Part model, mm, in its own coordinate system. A direction names the side the tool comes from. Coordinates: 2 decimals unless noted, no trailing zeros. Order: outer loops, then holes, each group sorted by start corner. A loop starts at its lowest first (then second) coordinate and runs counter-clockwise, first axis right, second up.
from build123d import *

# Parameters (mm, degrees)
PAD_DEPTH          = 4
SKETCH001_R        = 22.5
PAD001_DEPTH       = 2
SKETCH002_W        = 1.5
SKETCH002_H        = 5
POCKET_DEPTH       = 129.531389
POLARPATTERN_COUNT = 20


with BuildPart() as part:
    # Sketch → Pad (new body)
    with BuildSketch(Plane.XY):
        Polygon((-6.119913, 10.6), (-12.239826, 0), (-6.119913, -10.6), (6.119913, -10.6), (12.239826, 0), (6.119913, 10.6), align=None)
        Polygon((-4.965212, 8.6), (-9.930425, 0), (-4.965212, -8.6), (4.965212, -8.6), (9.930425, 0), (4.965212, 8.6), align=None, mode=Mode.SUBTRACT)
    extrude(amount=PAD_DEPTH)

    # Sketch001 (on Face13 of Pad) → Pad001 (join)
    with BuildSketch(Plane(origin=(0, 0, 0), x_dir=(1, 0, 0), z_dir=(0, 0, -1))):
        Circle(SKETCH001_R)
        Polygon((-6.119913, 10.6), (-12.239826, 0), (-6.119913, -10.6), (6.119913, -10.6), (12.239826, 0), (6.119913, 10.6), align=None, mode=Mode.SUBTRACT)
    extrude(amount=-PAD001_DEPTH)

    # Sketch002 (on Face2 of Pad001) → Pocket (cut, through all)
    with BuildSketch(Plane.XY.offset(2)):
        with Locations((0, 20)):
            Rectangle(SKETCH002_W, SKETCH002_H)
    pocket = extrude(amount=-POCKET_DEPTH, mode=Mode.SUBTRACT)

    # PolarPattern: Pocket ×20 about axis
    polarpattern_axis = Axis((0, 0, 0), (0, 0, 1))
    for i in range(1, POLARPATTERN_COUNT):
        add(pocket.rotate(polarpattern_axis, i * 360 / POLARPATTERN_COUNT), mode=Mode.SUBTRACT)


solid = part.part
Q1. Pin check, flat tips, straight feed: pin 1 Ø0.6 at (y, z) = (-19.5, 1) entering from -X; pin 2 Ø1 at (x, y) = (0, 12) entering from +Z; pin 3 Ø1.5 at (x, z) = (8.5, 2) entering from -Y. Stop position of each tip, or through.
Results list:
pin 1: stops at x = -11.73
pin 2: stops at z = 2
pin 3: stops at y = -21.12
Q2. Mould opens along X. For faces 1 (the face through (-12.34, 15.71, 1.01)), 2 (the face through (16.588, 11.125, 1.014)), 3 (the face through (17.5, 0, 1)), 4 (the face through (-17.5, 0, 1)) say: pulls with the +X half, pulls with the -X half, needs draft (parallel to the pull), parting line crosses it, or undercut.
Results list:
face 1: undercut
face 2: undercut
face 3: pulls with the +X half
face 4: pulls with the -X half
Q3. Wall check: line 1 along Y through (x, z) = (0, 2.4); line 2 along Y through (x, z) = (-17, 1.4); line 3 along X through (y, z) = (-14.5, 0.85). Give the ranges that are in metal, low to high.
Results list:
line 1: y = -10.6 to -8.6, 8.6 to 10.6
line 2: y = -14.74 to -13.28, -11.42 to -6.31, -4.74 to 4.74, 6.31 to 11.42, 13.28 to 14.74
line 3: x = -17.2 to -11.46, -9.82 to 9.82, 11.46 to 17.2
Q4. Cut at B-B on z = 3.15. Write the cut outline in (x, y), and give its area (3 significant figures).
Results list:
outline: (-12.24, 0) - (-6.12, -10.6) - (6.12, -10.6) - (12.24, 0) - (6.12, 10.6) - (-6.12, 10.6) - close; hole (-9.93, 0) - (-4.97, -8.6) - (4.97, -8.6) - (9.93, 0) - (4.97, 8.6) - (-4.97, 8.6) - close
area: 133 mm2
Q5. Cut at D-D on x = 3. Write the cut outline in (y, z).
Results list:
outline: (-22.3, 0) - (-8.6, 0) - (-8.6, 4) - (-10.6, 4) - (-10.6, 2) - (-22.3, 2) - close; (8.6, 0) - (22.3, 0) - (22.3, 2) - (10.6, 2) - (10.6, 4) - (8.6, 4) - close
Q6. Cut at C-C on x = -11.5. Write the cut outline in (y, z).
Results list:
outline: (-19.34, 0) - (-17.1, 0) - (-17.1, 2) - (-19.34, 2) - close; (-14.55, 0) - (14.55, 0) - (14.55, 2) - (1.28, 2) - (1.28, 4) - (-1.28, 4) - (-1.28, 2) - (-14.55, 2) - close; (17.1, 0) - (19.34, 0) - (19.34, 2) - (17.1, 2) - close
Q7. Cut at A-A on y = -2.5. Write the cut outline in (x, z), and give its area (3 significant figures).
Results list:
outline: (-22.36, 0) - (-8.49, 0) - (-8.49, 4) - (-10.8, 4) - (-10.8, 2) - (-22.36, 2) - close; (8.49, 0) - (22.36, 0) - (22.36, 2) - (10.8, 2) - (10.8, 4) - (8.49, 4) - close
area: 64.7 mm2
Q8. Which spindle directions (+Z, -Z, +X, -X, +Y, -Y) get a long thin tool onto all of the face, cutting with end or side? Do faces 5 (the face through (-20, -0.75, 1)), 6 (the face through (-9.14, 5.37, 2.99)), 7 (the face through (-0.75, 20, 1)), 8 (the face through (15.71, -12.34, 1.01)). Say none if no direction does.
Results list:
face 5: +Z, -Z, -X
face 6: +Z, -X, +Y
face 7: +Z, -Z, +Y
face 8: +Z, -Z
